from build123d import *

# Parameters (mm, degrees)
BOSS_EXTRUDE1_DEPTH = 3.075
SKETCH2_R           = 2.175
CUT_EXTRUDE2_DEPTH  = 6.35
BOSS_EXTRUDE2_DEPTH = 3.075
CUT_EXTRUDE3_DEPTH  = 10
FILLET1_R           = 10
CUT_EXTRUDE4_DEPTH  = 10


with BuildPart() as part:
    # Sketch1 → Boss-Extrude1 (new body)
    with BuildSketch(Plane(origin=(0, 0, 0), x_dir=(1, 0, 0), z_dir=(0, 1, 0))):
        with BuildLine():
            Line((-62.844661922, 8.700177936), (13.355338078, 8.700177936))
            ThreePointArc((13.355338078, 8.700177936), (19.705338078, 2.350177936), (13.355338078, -3.999822064))
            Line((13.355338078, -3.999822064), (-62.844661922, -3.999822064))
            ThreePointArc((-62.844661922, -3.999822064), (-69.194661922, 2.350177936), (-62.844661922, 8.700177936))
        make_face()
    extrude(amount=BOSS_EXTRUDE1_DEPTH)

    # Sketch2 → Cut-Extrude2 (cut)
    with BuildSketch(Plane(origin=(0, 3.075, 0), x_dir=(1, 0, 0), z_dir=(0, 1, 0))):
        with Locations(Location((-62.844661922, 2.350177936, 0), (0, 0, 270))):
            Circle(SKETCH2_R)
        with Locations(Location((-31.094661922, 2.350177936, 0), (0, 0, 270))):
            Circle(SKETCH2_R)
        with Locations(Location((1.555338078, 2.350177936, 0), (0, 0, 270))):
            Circle(SKETCH2_R)
    extrude(amount=-CUT_EXTRUDE2_DEPTH, mode=Mode.SUBTRACT)

    # Sketch3 → Boss-Extrude2 (add)
    with BuildSketch(Plane(origin=(0, 3.075, 0), x_dir=(1, 0, 0), z_dir=(0, 1, 0))):
        with BuildLine():
            Line((13.355338078, 8.700177936), (13.355338078, 2.350177936))
            Line((13.355338078, 2.350177936), (19.705338078, 2.350177936))
            Line((19.705338078, 2.350177936), (19.705338078, 9.999403669))
            ThreePointArc((19.705338078, 9.999403669), (19.189460997, 10.874403669), (18.174088078, 10.846618776))
            ThreePointArc((18.174088078, 10.846618776), (15.930319915, 9.401611756), (13.355338078, 8.700177936))
        make_face()
    extrude(amount=-BOSS_EXTRUDE2_DEPTH)

    # Sketch4 → Cut-Extrude3 (cut)
    with BuildSketch(Plane(origin=(0, 3.075, 0), x_dir=(1, 0, 0), z_dir=(0, 1, 0))):
        with BuildLine():
            Line((19.705338078, 9.999403669), (19.705338078, -6.000596331))
            Line((19.705338078, -6.000596331), (9.205338078, -6.000596331))
            ThreePointArc((9.205338078, -6.000596331), (16.836220051, 0.436949875), (19.705338078, 9.999403669))
        make_face()
    extrude(amount=-CUT_EXTRUDE3_DEPTH, mode=Mode.SUBTRACT)

    # Fillet1
    fillet1_edges = [part.edges().sort_by_distance(p)[0] for p in [
        (12.654174153, 1.5375, 3.999822064),
    ]]
    fillet(fillet1_edges, radius=FILLET1_R)

    # Sketch5 → Cut-Extrude4 (cut)
    with BuildSketch(Plane(origin=(0, 3.075, 0), x_dir=(1, 0, 0), z_dir=(0, 1, 0))):
        Polygon((-4.314661922, 8.700177936), (-0.914661922, 8.700177936), (-1.614661922, 7.306047383), (-3.614661922, 7.306047383), align=None)
        Polygon((-9.814661922, 8.700177936), (-9.114661922, 7.306047383), (-7.114661922, 7.306047383), (-6.414661922, 8.700177936), align=None)
        Polygon((1.185338078, 8.700177936), (4.585338078, 8.700177936), (3.885338078, 7.306047383), (1.885338078, 7.306047383), align=None)
        Polygon((6.685338078, 8.700177936), (10.085338078, 8.700177936), (9.385338078, 7.306047383), (7.385338078, 7.306047383), align=None)
        Polygon((-15.314661922, 8.700177936), (-11.914661922, 8.700177936), (-12.614661922, 7.306047383), (-14.614661922, 7.306047383), align=None)
        Polygon((-20.814661922, 8.700177936), (-17.414661922, 8.700177936), (-18.114661922, 7.306047383), (-20.114661922, 7.306047383), align=None)
        Polygon((-26.314661922, 8.700177936), (-22.914661922, 8.700177936), (-23.614661922, 7.306047383), (-25.614661922, 7.306047383), align=None)
    extrude(amount=-CUT_EXTRUDE4_DEPTH, mode=Mode.SUBTRACT)


solid = part.part
Input: part model. Units: mm. Frame: model coordinates. A direction names the side the tool comes from. Round coordinates to 2 decimals unless told otherwise and drop trailing zeros. Order: outer loops, then holes, each group sorted by start corner. A loop starts at its lowest first (then second) coordinate and runs counter-clockwise, first axis right, second up. Notation, with made-up numbers: (67, 66.25) - (109, 66.25) arc R8 cw to (109, 73.25) - close; hole circle Ø7 at (44, 8.5). An arc over 180 degrees is marked (long way). Answer as a JSON object with one key per item and string values. Group by question number.
(1) Cut plane C-C (z = 2.5). Return loops of the section in (x, y) (3 decimals).
(2) Cut plane B-B (x = -49.5). Return loops of the section in (y, z) (3 decimals).
(3) Draft query along X for faces 4 (the face through (-3.96, 1.56, -7.99)), 5 (the face through (-45, 2, -8.7)), 6 (the face through (18.978, 1.559, -5.045)). Return one class per face: released by +X, released by -X, zero draft, split by the parting line, or undercut.
(4) Material intervals for probe 1 along X at (y, z) = (1.8, -2.5); probe 2 along X at (y, z) = (1.65, -3.5); probe 3 along Z at (x, y) = (-10, 0.95), sorted ascending. Write a range as from..to.
(5) Cut plane A-A (z = -2.75). Return loops of the section in (x, y) (3 decimals), then the cut area to 3 significant figures.
(6) Reachability of faces 1 (the face through (-8, 2, -7.306)), 2 (the face through (-24, 3.075, -2)), 3 (the face through (6, 2, -8.7)) from +Z, -Z, +X, -X, +Y, -Y: full face, straight path, thin tool, end or side. Return the list, or none.
(7) Cut plane D-D (y = 0.6). Count the separate pieces of the cut face and the enclosed holes in it, then the cut area to 3 significant figures.
(8) Pin query (flat end, axial travel): P1, Ø1, axis at y = 1, z = -1.5, coming from the -X side (3 decimals); P2, Ø1, axis at x = -8.5, y = 2, coming from the -Z side; P3, Ø1.1, axis at x = -16, y = 2, coming from the -Z side. Return the tip coordinate at first contact, or that it passes through.
Here are the results:
{
 "1": {"outline": "(-66.943, 0) - (13.793, 0) - (13.793, 3.075) - (-66.943, 3.075) - close"},
 "2": {"outline": "(0, -8.7) - (3.075, -8.7) - (3.075, 4) - (0, 4) - close"},
 "3": {"face 4": "undercut", "face 5": "zero draft", "face 6": "released by +X"},
 "4": {"probe 1": "x = -69.19..-65.01, -60.67..-33.26, -28.92..-0.61, 3.73..18", "probe 2": "x = -69.09..-64.69, -61..-32.94, -29.25..-0.29, 3.4..18.44", "probe 3": "z = -8.7..4"},
 "5": {"outline": "(-69.182, 0) - (-64.983, 0) - (-64.983, 3.075) - (-69.182, 3.075) - close; (-60.707, 0) - (-33.233, 0) - (-33.233, 3.075) - (-60.707, 3.075) - close; (-28.957, 0) - (-0.583, 0) - (-0.583, 3.075) - (-28.957, 3.075) - close; (3.693, 0) - (18.115, 0) - (18.115, 3.075) - (3.693, 3.075) - close", "area": "229 mm^2"},
 "6": {"face 1": "-Z, +Y, -Y", "face 2": "+Z, -Z, +X, -X, +Y", "face 3": "-Z, -X, +Y, -Y"},
 "7": {"separate pieces": "1", "enclosed holes": "3", "area": "1,020 mm^2"},
 "8": {"P1": "stops at x = -69.185", "P2": "stops at z = -7.31", "P3": "stops at z = -8.7"}
}
